Design review of the part built by this model. Coordinates are the model's own, in mm. Face numbers are marked on the shaded views. A direction names the side the tool comes from. Give positions to 0.01 mm unless a question says otherwise; leave off trailing zeros. Write each loop counter-clockwise with the first axis right and the second up, starting at its lowest first coordinate (ties: lowest second). Pieces come first, ordered by that corner, then holes. Notation, with made-up numbers: (23, 11) -> (60, 11) arc R25 ccw to (60, 48) -> close; hole circle Ø3 at (88, 26.5). An arc over 180 degrees is marked (long way). Return JSON: item names as keys, results as strings. Group by question number.
from build123d import *

# Parameters (mm, degrees)
SKETCH_W            = 165
SKETCH_H            = 165
PAD_DEPTH           = 65
SKETCH002_W         = 152
SKETCH002_H         = 152
POCKET_DEPTH        = 6.5
SKETCH003_W         = 145
SKETCH003_H         = 145
POCKET001_DEPTH     = 55
SKETCH005_W         = 156.6
SKETCH005_H         = 3.5
POCKET003_DEPTH     = 160
POCKET004_DEPTH     = 165.001
LINEARPATTERN_COUNT = 4
LINEARPATTERN_PITCH = 6.666667
SKETCH008_W         = 10
SKETCH008_H         = 10
POCKET005_DEPTH     = 32
POCKET006_DEPTH     = 9
SKETCH013_W         = 50.5
SKETCH013_H         = 5.4
POCKET007_DEPTH     = 7
CHAMFER_ANGLE       = 30
CHAMFER_SIZE        = 12
CHAMFER001_ANGLE    = 30
CHAMFER001_SIZE     = 12
POCKET008_DEPTH     = 1.001


with BuildPart() as part:
    # Sketch → Pad (new body)
    with BuildSketch(Plane.XY):
        Rectangle(SKETCH_W, SKETCH_H)
    extrude(amount=PAD_DEPTH)

    # Sketch002 (on Face6 of Pad) → Pocket (cut)
    with BuildSketch(Plane.XY.offset(65)):
        Rectangle(SKETCH002_W, SKETCH002_H)
    extrude(amount=-POCKET_DEPTH, mode=Mode.SUBTRACT)

    # Sketch003 (on Face11 of Pocket) → Pocket001 (cut)
    with BuildSketch(Plane.XY.offset(58.5)):
        Rectangle(SKETCH003_W, SKETCH003_H)
    extrude(amount=-POCKET001_DEPTH, mode=Mode.SUBTRACT)

    # Sketch005 → Pocket003 (cut)
    with BuildSketch(Plane.XZ.offset(82.5)):
        with Locations((0, 60.25)):
            Rectangle(SKETCH005_W, SKETCH005_H)
    extrude(amount=-POCKET003_DEPTH, mode=Mode.SUBTRACT)

    # Sketch007 (on Face2 of Pocket003) → Pocket004 (cut, through all)
    with BuildSketch(Plane(origin=(-82.5, 0, 0), x_dir=(0, -1, 0), z_dir=(-1, 0, 0))):
        with BuildLine():
            ThreePointArc((58, 15), (60, 13), (62, 15))
            Line((62, 15), (62, 31))
            ThreePointArc((62, 31), (60, 33), (58, 31))
            Line((58, 15), (58, 31))
        make_face()
    pocket004 = extrude(amount=-POCKET004_DEPTH, mode=Mode.SUBTRACT)

    # LinearPattern: Pocket004 ×4
    with Locations(*[(0, i * LINEARPATTERN_PITCH, 0) for i in range(1, LINEARPATTERN_COUNT)]):
        add(pocket004, mode=Mode.SUBTRACT)

    # Sketch008 (on Face10 of LinearPattern) → Pocket005 (cut)
    with BuildSketch(Plane(origin=(0, 82.5, 0), x_dir=(-1, 0, 0), z_dir=(0, 1, 0))):
        with Locations((0, 5)):
            Rectangle(SKETCH008_W, SKETCH008_H)
    extrude(amount=-POCKET005_DEPTH, mode=Mode.SUBTRACT)

    # Sketch012 (on Face53 of Pocket005) → Pocket006 (cut)
    with BuildSketch(Plane.XZ.offset(-72.5)):
        with BuildLine():
            ThreePointArc((-14.98, 43.25), (-22.814744, 33.125), (-14.98, 23))
            Line((-14.98, 23), (15.02, 23))
            ThreePointArc((15.02, 23), (22.824854, 33.125), (15.02, 43.25))
            Line((-14.98, 43.25), (15.02, 43.25))
        make_face()
    extrude(amount=-POCKET006_DEPTH, mode=Mode.SUBTRACT)

    # Sketch013 (on Face53 of Pocket006) → Pocket007 (cut)
    with BuildSketch(Plane.XZ.offset(-72.5)):
        with Locations((0, 33.25)):
            Rectangle(SKETCH013_W, SKETCH013_H)
    extrude(amount=-POCKET007_DEPTH, mode=Mode.SUBTRACT)

    # Chamfer
    chamfer_edges = [part.edges().sort_by_distance(p)[0] for p in [
        (-25.25, 72.5, 33.25),
    ]]
    chamfer_side = part.faces().sort_by_distance((0, 72.5, 56.949194))[0]
    chamfer(chamfer_edges, length=CHAMFER_SIZE, angle=CHAMFER_ANGLE, reference=chamfer_side)

    # Chamfer001
    chamfer001_edges = [part.edges().sort_by_distance(p)[0] for p in [
        (25.25, 72.5, 33.25),
    ]]
    chamfer001_side = part.faces().sort_by_distance((-31.25, 72.5, 37.500806))[0]
    chamfer(chamfer001_edges, length=CHAMFER001_SIZE, angle=CHAMFER001_ANGLE, reference=chamfer001_side)

    # Sketch014 (on Face21 of Chamfer001) → Pocket008 (cut, through all)
    with BuildSketch(Plane.XZ.offset(-81.5)):
        with BuildLine():
            Line((12.35, 39.36), (-12.35, 39.36))
            ThreePointArc((-12.35, 39.36), (-18.455, 33.255), (-12.35, 27.15))
            Line((-12.35, 27.15), (12.35, 27.15))
            ThreePointArc((12.35, 27.15), (18.455, 33.255), (12.35, 39.36))
        make_face()
    extrude(amount=-POCKET008_DEPTH, mode=Mode.SUBTRACT)


solid = part.part
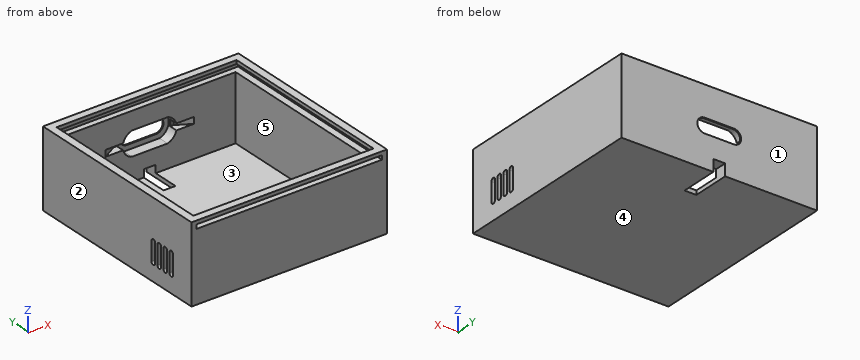
Q1. Mouldability with a two-part tool opening along Y and no side actions: class the marked faces 1, 2 and 3 as +Y half, -Y half, draft (parallel to the pull), parting line (faces both ways), or undercut.
Q2. Take a section at B-B, the plane y = 66. Give the boundary of the cut face in (x, z), plus the area to 3 significant figures.
Q3. Insertion check: pin 1 (1.8 mm diameter, centred on x = 1, z = 1.5, fed in from +Y); pin 2 (12 mm diameter, centred on x = 32, y = 27.5, fed in from +Z). Each pin has a flat end and moves straight along its axis. Give the tip position at first contact, or say it passes through.
Q4. Take a section at A-A, the plane x = 47. Give the boundary of the cut face in (y, z).
Q5. For L1, parallel to X at y = -43, z = 24.5; L2, parallel to Y at x = -22.5, z = 32, list the stretches that pass through material, from the lowest coordinate up. Write a range as from..to.
Q6. Take a section at C-C, the plane z = 45.5. Give the boundary of the cut face in (x, y).
Q7. Tool access review of the marked faces 4 and 5: name each direction out of +Z, -Z, +X, -X, +Y, -Y from which nothing blocks a thin tool from reaching the whole face with its end or side.
Q8. Take a section at D-D, the plane y = -69.5. Give the boundary of the cut face in (x, z), plus the area to 3 significant figures.
Final values:
{
 "1": {"face 1": "+Y half", "face 2": "draft", "face 3": "undercut"},
 "2": {"outline": "(-82.5, 0) -> (-5, 0) -> (-5, 3.5) -> (-72.5, 3.5) -> (-72.5, 58.5) -> (-78.3, 58.5) -> (-78.3, 62) -> (-76, 62) -> (-76, 65) -> (-82.5, 65) -> close; (5, 0) -> (82.5, 0) -> (82.5, 65) -> (76, 65) -> (76, 62) -> (78.3, 62) -> (78.3, 58.5) -> (72.5, 58.5) -> (72.5, 3.5) -> (5, 3.5) -> close", "area": "1,710 mm²"},
 "3": {"pin 1": "stops at y = 50.5", "pin 2": "stops at z = 3.5"},
 "4": {"outline": "(-82.5, 0) -> (82.5, 0) -> (82.5, 65) -> (76, 65) -> (76, 62) -> (77.5, 62) -> (77.5, 58.5) -> (72.5, 58.5) -> (72.5, 3.5) -> (-72.5, 3.5) -> (-72.5, 58.5) -> (-82.5, 58.5) -> close; (-82.5, 62) -> (-76, 62) -> (-76, 65) -> (-82.5, 65) -> close"},
 "5": {"L1": "x = -82.5..-72.5, 72.5..82.5", "L2": "y = -82.5..-72.5, 81.5..82.5"},
 "6": {"outline": "(-82.5, -82.5) -> (82.5, -82.5) -> (82.5, 82.5) -> (-82.5, 82.5) -> close; hole (-72.5, -72.5) -> (72.5, -72.5) -> (72.5, 72.5) -> (-72.5, 72.5) -> close"},
 "7": {"face 4": "-Z, +X, -X, +Y, -Y", "face 5": "+Z"},
 "8": {"outline": "(-82.5, 0) -> (82.5, 0) -> (82.5, 65) -> (76, 65) -> (76, 62) -> (78.3, 62) -> (78.3, 58.5) -> (72.5, 58.5) -> (72.5, 3.5) -> (-72.5, 3.5) -> (-72.5, 58.5) -> (-78.3, 58.5) -> (-78.3, 62) -> (-76, 62) -> (-76, 65) -> (-82.5, 65) -> close", "area": "1,750 mm²"}
}
